```python
from build123d import *

# Parameters (mm, degrees)
SKETCH1_W           = 465
SKETCH1_H           = 90
SKETCH1_R           = 2.55
BOSS_EXTRUDE1_DEPTH = 2.2479
CUT_EXTRUDE1_REACH  = 6.496


with BuildPart() as part:
    # Sketch1 → Boss-Extrude1 (new body, symmetric)
    with BuildSketch(Plane.XY):
        Rectangle(SKETCH1_W, SKETCH1_H)
        with Locations((-222.5, 35)):
            Circle(SKETCH1_R, mode=Mode.SUBTRACT)
        with Locations((-222.5, -35)):
            Circle(SKETCH1_R, mode=Mode.SUBTRACT)
        with Locations((0, 35)):
            Circle(SKETCH1_R, mode=Mode.SUBTRACT)
        with Locations((-114.975, 35)):
            Circle(SKETCH1_R, mode=Mode.SUBTRACT)
        with Locations((222.5, -35)):
            Circle(SKETCH1_R, mode=Mode.SUBTRACT)
        with Locations((222.5, 35)):
            Circle(SKETCH1_R, mode=Mode.SUBTRACT)
        with Locations((114.975, 35)):
            Circle(SKETCH1_R, mode=Mode.SUBTRACT)
    extrude(amount=BOSS_EXTRUDE1_DEPTH, both=True)

    # Sketch2 → Cut-Extrude1 (cut, up to next)
    with BuildSketch(Plane.XY.offset(2.2479), mode=Mode.PRIVATE) as cut_extrude1_sk1:
        Polygon((-159.938544521, -8), (-170.794476725, 22.5), (-200.205523275, 22.5), (-211.061455479, -8), (-200.205523275, -38.5), (-170.794476725, -38.5), align=None)
    cut_extrude1_tool1 = extrude(cut_extrude1_sk1.sketch, amount=-CUT_EXTRUDE1_REACH, mode=Mode.PRIVATE) & part.part
    add(cut_extrude1_tool1.solids().sort_by_distance((-185.5, -8, 2.2479))[0], mode=Mode.SUBTRACT)


solid = part.part
```
Check sheet for the modelled part. Datum: model origin and axes. Units: mm. A direction names the side the tool comes from. Give positions to 0.01 mm unless a question says otherwise; leave off trailing zeros. Loops run counter-clockwise (first coordinate to the right, second up) from the corner with the lowest first, then second, coordinate; pieces in that order, holes last. Notation, with made-up numbers: (55, -39.5) - (69, -39.5) arc R10 cw to (69, -20.5) - close; hole circle Ø7 at (54, 85.5). An arc over 180 degrees is marked (long way). One line per question, with ' | ' between items. Start each with the question number.
1. Set-up check for faces 1 (the flat face through (-3, 1, 2.248)), 2 (the flat face through (-205.56, 7.46, 0.03)): record each of +Z, -Z, +X, -X, +Y, -Y from which the full face is reachable in a straight line by a thin tool's end or side.
2. Cross-section at B-B, the plane y = -18. Enter the section's corners in (x, z).
3. Cross-section at C-C, the plane y = 15.5. Enter the section's corners in (x, z), plus the area to 3 significant figures.
4. Draft check along Y on faces 3 (the flat face through (-165.29, 7.04, 0.03)), 4 (the flat face through (-205.71, -23.04, 0.03)), 5 (the flat face through (-3, 1, -2.248)). Enter one of: released by +Y, released by -Y, zero draft, split by the parting line, or undercut.
5. Cross-section at A-A, the plane z = -1.3. Give the number of separate pieces and of enclosed holes in the cut face, plus the area to 3 significant figures.
6. Material ranges on line 1 along Y through (x, z) = (222.5, -1.2); line 2 along Y through (x, z) = (-173.5, -1.25); line 3 along Y through (x, z) = (0, 0.65), recorded low to high. Write a range as [from, to].
Check result:
1) face 1: +Z, +X, -X, +Y, -Y | face 2: +Z, -Z
2) outline: (-232.5, -2.25) - (-207.5, -2.25) - (-207.5, 2.25) - (-232.5, 2.25) - close; (-163.5, -2.25) - (232.5, -2.25) - (232.5, 2.25) - (-163.5, 2.25) - close
3) outline: (-232.5, -2.25) - (-202.7, -2.25) - (-202.7, 2.25) - (-232.5, 2.25) - close; (-168.3, -2.25) - (232.5, -2.25) - (232.5, 2.25) - (-168.3, 2.25) - close | area: 1,940 mm2
4) face 3: undercut | face 4: undercut | face 5: zero draft
5) separate pieces: 1 | enclosed holes: 8 | area: 39,300 mm2
6) line 1: y = [-45, -37.55], [-32.45, 32.45], [37.55, 45] | line 2: y = [-45, -38.5], [22.5, 45] | line 3: y = [-45, 32.45], [37.55, 45]
